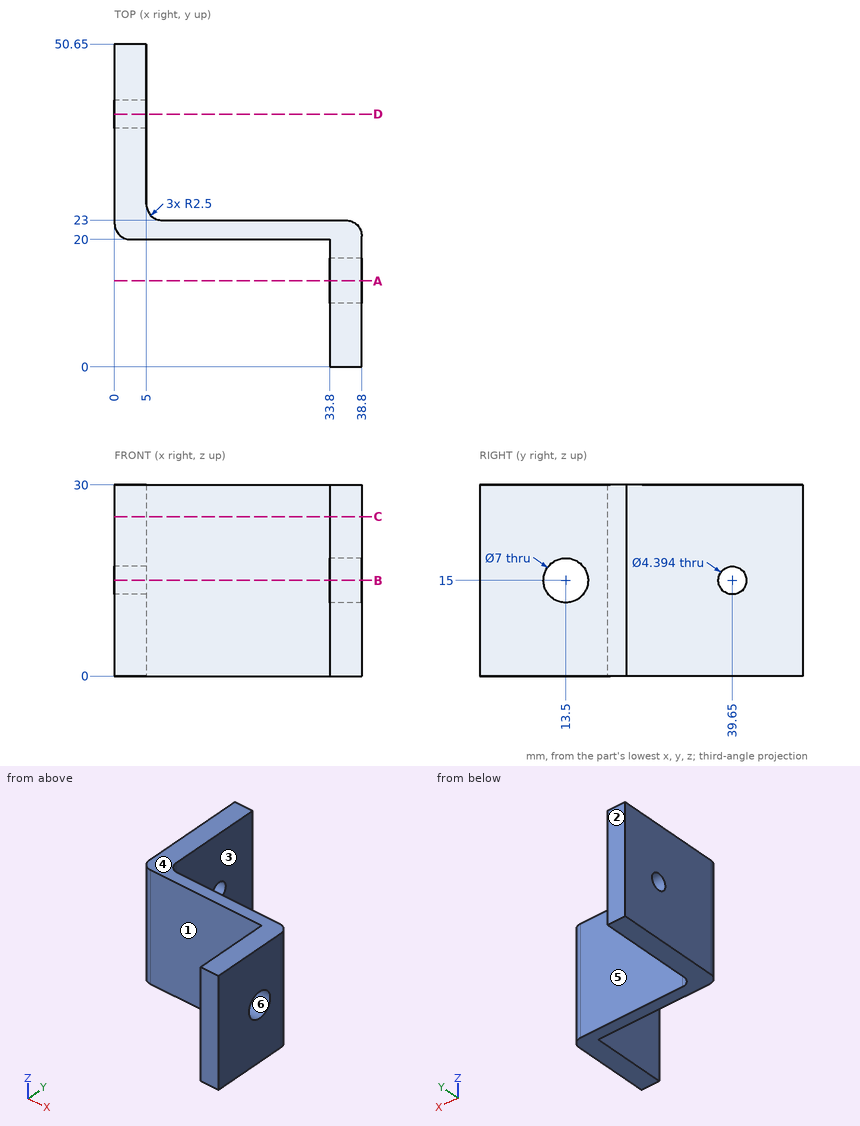
Input: dimensioned drawing with shaded views. Units: mm. Origin: part minimum x, y, z. A direction names the side the tool comes from. Give positions to 0.01 mm unless a question says otherwise; leave off trailing zeros. Order: outer loops, then holes, each group sorted by start corner. A loop starts at its lowest first (then second) coordinate and runs counter-clockwise, first axis right, second up.
(1) Pull-direction query (Y, two-part tool) for the marked faces 4, 5 and 6; classes: +Y half, -Y half, draft (parallel to the pull), parting line (faces both ways), or undercut.
(2) Contact query for flat-ended pins moving along their axis: P1, Ø6, axis at x = 8.5, y = 27, coming from the +Z side; P2, Ø6, axis at y = 21, z = 21.5, coming from the +X side; P3, Ø8.5, axis at x = 16, z = 8, coming from the +Y side; P4, Ø16, axis at y = 8, z = 9, coming from the -X side. Output: stop coordinate, or through.
(3) Section query C-C (z = 25). Return the cut outline in (x, y), plus the area to 3 significant figures.
(4) Material intervals for line 1 along Y through (x, z) = (35.1, 15); line 2 along Z through (x, y) = (3.65, 39.65); line 3 along X through (y, z) = (39, 19.5), sorted ascending.
(5) Section query D-D (y = 39.65). Return the cut outline in (x, z).
(6) Section query B-B (z = 15). Return the cut outline in (x, y).
(7) Access query for the marked faces 1, 2 and 3. Directions: +Z, -Z, +X, -X, +Y, -Y. A direction counts if a zero-diameter tool reaches every point of the face in a straight line with its end or side. Return the directions, or none.
(8) Section query A-A (y = 13.5). Return the cut outline in (x, z), plus the area to 3 significant figures.
Outcome:
1. face 4: draft
1. face 5: +Y half
1. face 6: undercut
2. P1: passes through
2. P2: stops at x = 38.8
2. P3: stops at y = 23
2. P4: stops at x = 33.8
3. outline: (0, 22.5) arc R2.5 ccw to (2.5, 20) - (33.8, 20) - (33.8, 0) - (38.8, 0) - (38.8, 20.5) arc R2.5 ccw to (36.3, 23) - (7.5, 23) arc R2.5 cw to (5, 25.5) - (5, 50.65) - (0, 50.65) - close
3. area: 353 mm2
4. line 1: y = 0 to 10, 17 to 23
4. line 2: z = 0 to 12.8, 17.2 to 30
4. line 3: x = 0 to 5
5. outline: (0, 0) - (5, 0) - (5, 12.8) - (0, 12.8) - close; (0, 17.2) - (5, 17.2) - (5, 30) - (0, 30) - close
6. outline: (0, 22.5) arc R2.5 ccw to (2.5, 20) - (33.8, 20) - (33.8, 17) - (38.8, 17) - (38.8, 20.5) arc R2.5 ccw to (36.3, 23) - (7.5, 23) arc R2.5 cw to (5, 25.5) - (5, 37.45) - (0, 37.45) - close; (0, 41.85) - (5, 41.85) - (5, 50.65) - (0, 50.65) - close; (33.8, 0) - (38.8, 0) - (38.8, 10) - (33.8, 10) - close
7. face 1: +Z, -Z, -X, -Y
7. face 2: +Z, -Z, +X, -X, +Y
7. face 3: +Z, -Z, +X, +Y
8. outline: (33.8, 0) - (38.8, 0) - (38.8, 11.5) - (33.8, 11.5) - close; (33.8, 18.5) - (38.8, 18.5) - (38.8, 30) - (33.8, 30) - close
8. area: 115 mm2
